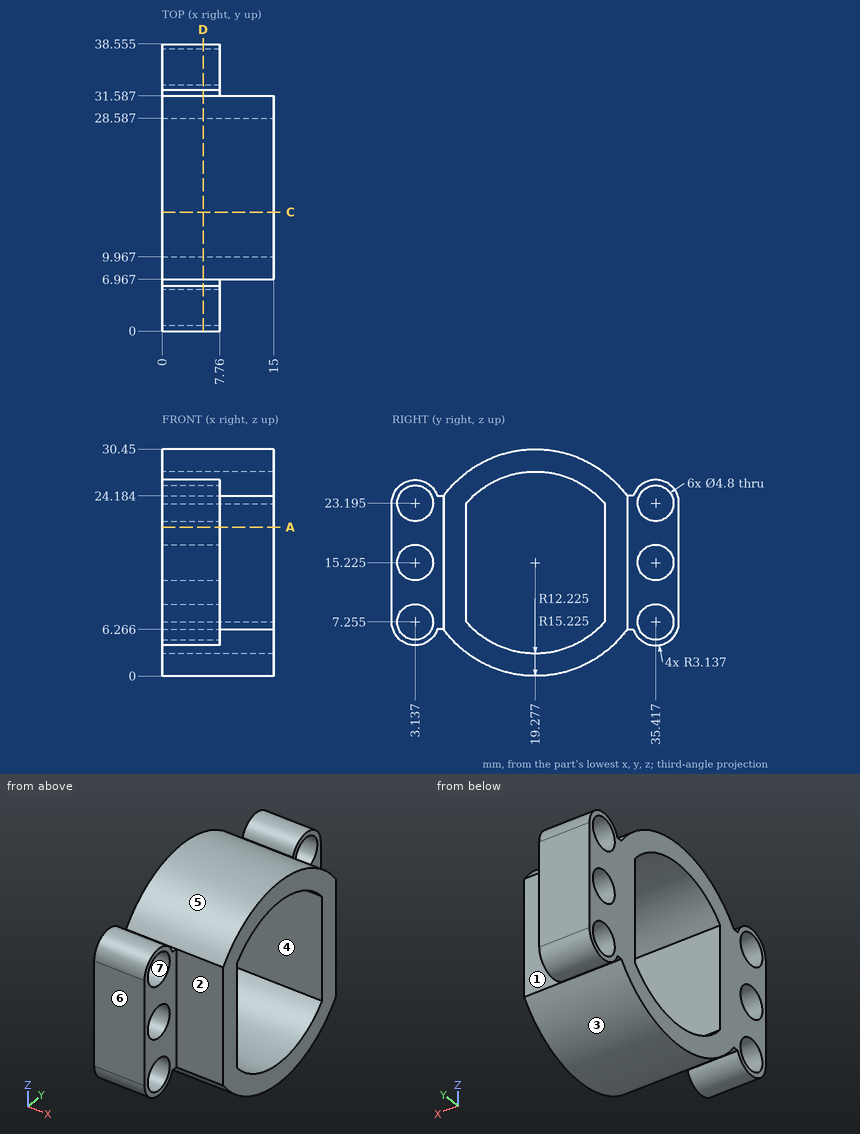
Answer from the drawing. Dimensions are ordinates in mm from the lowest x, y and z of the part. A direction names the side the tool comes from. Coordinates: 2 decimals unless noted, no trailing zeros. Order: outer loops, then holes, each group sorted by start corner. A loop starts at its lowest first (then second) coordinate and runs counter-clockwise, first axis right, second up. Notation, with made-up numbers: (51.5, 32) - (84.5, 32) arc R12 ccw to (84.5, 36) - close; hole circle Ø2 at (-2, -14). An arc over 180 degrees is marked (long way). Put each result on its own line as item: value. Start each with the question number.
1) For the marked faces 1, 2, 3 and 4, determine the directions among +Z, -Z, +X, -X, +Y, -Y from which every point of the face is accessible in a straight line to the end or side of a thin tool.
2) For a pull along Z with two mould halves and no side action, classify the marked faces 5, 6 and 7 as released by +Z, released by -Z, zero draft, split by the parting line, or undercut.
3) Find section A-A (z = 20). Give the vertices of the cut face in (x, y) (1 decimal).
4) Find the intervals of material crossed by line 1 (Y direction, x = 12.5, z = 9.5); line 2 (Z direction, x = 1.75, y = 35.5); line 3 (Y direction, x = 1, z = 17) (1 decimal), in increasing order. Write a range as from..to.
5) Find section D-D (x = 5.5). State how many separate pieces and enclosed holes the cut face has, plus the area to 3 significant figures.
6) Find section C-C (y = 16). Give the vertices of the cut face in (x, z).
7) Flat-ended cylindrical pins translate along their axes: pin 1 (1 mm diameter, centred on x = 10.5, y = 28, fed in from -Z); pin 2 (5.5 mm diameter, centred on y = 35.42, z = 7.26, fed in from +X); pin 3 (2 mm diameter, centred on x = 11.5, z = 16, fed in from +Y). Find the tip coordinate at first contact, or state that the pin passes through.
Results list:
1. face 1: +Z, -Z, +X, +Y
1. face 2: +Z, -Z, +X, -Y
1. face 3: -Z, +X, -X
1. face 4: +X, -X
2. face 5: released by +Z
2. face 6: zero draft
2. face 7: undercut
3. outline: (0, 0) - (7.8, 0) - (7.8, 7) - (15, 7) - (15, 10) - (0, 10) - close; (0, 28.6) - (15, 28.6) - (15, 31.6) - (7.8, 31.6) - (7.8, 38.6) - (0, 38.6) - close
4. line 1: y = 6.97..9.97, 28.59..31.59
4. line 2: z = 4.12..4.86, 9.65..12.83, 17.62..20.8, 25.59..26.33
4. line 3: y = 0..1.5, 4.8..10, 28.6..33.8, 37..38.6
5. separate pieces: 1
5. enclosed holes: 7
5. area: 429 mm^2
6. outline: (0, 0.36) - (15, 0.36) - (15, 3.45) - (0, 3.45) - close; (0, 27) - (15, 27) - (15, 30.09) - (0, 30.09) - close
7. pin 1: stops at z = 2.41
7. pin 2: stops at x = 7.76
7. pin 3: stops at y = 31.59
